Part model, mm, in its own coordinate system. A direction names the side the tool comes from. Round coordinates to 2 decimals unless told otherwise and drop trailing zeros. Order: outer loops, then holes, each group sorted by start corner. A loop starts at its lowest first (then second) coordinate and runs counter-clockwise, first axis right, second up. Notation, with made-up numbers: (-15.75, 66.5) - (2.25, 66.5) arc R35 cw to (2.25, 100.5) - close; hole circle Ø11 at (78, -14.5). An arc over 180 degrees is marked (long way). Answer as a JSON object with one key per item and string values.
```python
from build123d import *

# Parameters (mm, degrees)
SKETCH_1_W          = 33
SKETCH_1_H          = 62
EXTRUDE_1_DEPTH     = 8
SKETCH_2_W          = 15
SKETCH_2_H          = 10
CUT_EXTRUDE_1_DEPTH = 37.017356927
SKETCH_3_R          = 1.5
CUT_EXTRUDE_2_DEPTH = 37.017356927
SKETCH_4_R          = 1.5
CUT_EXTRUDE_3_DEPTH = 46.97825573
FILLET_2_R          = 1
SKETCH_5_R          = 1.5
CUT_EXTRUDE_4_DEPTH = 37.017356927
SKETCH_7_W          = 15
SKETCH_7_H          = 10
CUT_EXTRUDE_5_DEPTH = 37.017356927
FILLET_3_R          = 3
SKETCH_8_R          = 3.5
SKETCH_8_R_2        = 3
CUT_EXTRUDE_6_DEPTH = 3.5


with BuildPart() as part:
    # 草图1 → 凸台-拉伸1 (new body)
    with BuildSketch(Plane.XY):
        Rectangle(SKETCH_1_W, SKETCH_1_H)
    extrude(amount=EXTRUDE_1_DEPTH)

    # 草图2 → 切除-拉伸1 (cut, through all)
    with BuildSketch(Plane.XY.offset(8)):
        with Locations((0, 26)):
            Rectangle(SKETCH_2_W, SKETCH_2_H)
        with Locations((0, -26)):
            Rectangle(SKETCH_2_W, SKETCH_2_H)
    extrude(amount=-CUT_EXTRUDE_1_DEPTH, mode=Mode.SUBTRACT)

    # 草图3 → 切除-拉伸2 (cut, through all)
    with BuildSketch(Plane.XY.offset(8)):
        with Locations((11.5, 13)):
            Circle(SKETCH_3_R)
        with Locations((11.5, 21)):
            Circle(SKETCH_3_R)
        with Locations(Location((11.5, -21, 0), (0, 0, 180))):
            Circle(SKETCH_3_R)
        with Locations(Location((11.5, -13, 0), (0, 0, 180))):
            Circle(SKETCH_3_R)
        with Locations((-11.5, -13)):
            Circle(SKETCH_3_R)
        with Locations((-11.5, -21)):
            Circle(SKETCH_3_R)
        with Locations(Location((-11.5, 21, 0), (0, 0, 180))):
            Circle(SKETCH_3_R)
        with Locations(Location((-11.5, 13, 0), (0, 0, 180))):
            Circle(SKETCH_3_R)
    extrude(amount=-CUT_EXTRUDE_2_DEPTH, mode=Mode.SUBTRACT)

    # 草图4 → 切除-拉伸3 (cut, through all)
    with BuildSketch(Plane.ZY.offset(16.5)):
        with Locations((5, 27)):
            Circle(SKETCH_4_R)
        with Locations(Location((5, -27, 0), (0, 0, 180))):
            Circle(SKETCH_4_R)
    extrude(amount=-CUT_EXTRUDE_3_DEPTH, mode=Mode.SUBTRACT)

    # 圆角2
    fillet_2_edges = [part.edges().sort_by_distance(p)[0] for p in [
        (7.5, 21, 4),
        (-7.5, 21, 4),
        (-7.5, -21, 4),
        (7.5, -21, 4),
    ]]
    fillet(fillet_2_edges, radius=FILLET_2_R)

    # 草图5 → 切除-拉伸4 (cut, through all)
    with BuildSketch(Plane(origin=(0, 0, 0), x_dir=(-1, 0, 0), z_dir=(0, 0, -1))):
        Circle(SKETCH_5_R)
        with Locations((0, 18)):
            Circle(SKETCH_5_R)
        with Locations(Location((0, -18, 0), (0, 0, 180))):
            Circle(SKETCH_5_R)
    extrude(amount=-CUT_EXTRUDE_4_DEPTH, mode=Mode.SUBTRACT)

    # 草图7 → 切除-拉伸5 (cut, through all)
    with BuildSketch(Plane(origin=(0, 0, 0), x_dir=(-1, 0, 0), z_dir=(0, 0, -1))):
        with Locations((0, 9)):
            Rectangle(SKETCH_7_W, SKETCH_7_H)
        with Locations((0, -9)):
            Rectangle(SKETCH_7_W, SKETCH_7_H)
    extrude(amount=-CUT_EXTRUDE_5_DEPTH, mode=Mode.SUBTRACT)

    # 圆角3
    fillet_3_edges = [part.edges().sort_by_distance(p)[0] for p in [
        (-7.5, 14, 4),
        (-7.5, 4, 4),
        (7.5, 4, 4),
        (7.5, 14, 4),
        (7.5, -14, 4),
        (7.5, -4, 4),
        (-7.5, -4, 4),
        (-7.5, -14, 4),
    ]]
    fillet(fillet_3_edges, radius=FILLET_3_R)

    # 草图8 → 切除-拉伸6 (cut)
    with BuildSketch(Plane(origin=(0, 0, 0), x_dir=(-1, 0, 0), z_dir=(0, 0, -1))):
        with Locations((11.5, 21)):
            Circle(SKETCH_8_R)
        with Locations((-11.5, 21)):
            Circle(SKETCH_8_R)
        with Locations((-11.5, -21)):
            Circle(SKETCH_8_R)
        with Locations((11.5, -21)):
            Circle(SKETCH_8_R)
        Circle(SKETCH_8_R_2)
    extrude(amount=-CUT_EXTRUDE_6_DEPTH, mode=Mode.SUBTRACT)


solid = part.part
```
Item 1: Cut at B-B (y = 0). Write the cut outline in (x, z).
Taken from the geometry:
{"outline": "(-16.5, 0) - (-3, 0) - (-3, 3.5) - (-1.5, 3.5) - (-1.5, 8) - (-16.5, 8) - close; (1.5, 3.5) - (3, 3.5) - (3, 0) - (16.5, 0) - (16.5, 8) - (1.5, 8) - close"}
Item 2: Cut at C-C (y = 27). Write the cut outline in (x, z), plus the area to 3 significant figures.
Taken from the geometry:
{"outline": "(-16.5, 0) - (-7.5, 0) - (-7.5, 3.5) - (-16.5, 3.5) - close; (-16.5, 6.5) - (-7.5, 6.5) - (-7.5, 8) - (-16.5, 8) - close; (7.5, 0) - (16.5, 0) - (16.5, 3.5) - (7.5, 3.5) - close; (7.5, 6.5) - (16.5, 6.5) - (16.5, 8) - (7.5, 8) - close", "area": "90.0 mm2"}
Item 3: Cut at A-A (x = -11.5). State how many separate pieces and enclosed holes the cut face has, plus the area to 3 significant figures.
Taken from the geometry:
{"separate pieces": "5", "enclosed holes": "2", "area": "358 mm2"}
Item 4: Probe L1, parallel to Y at x = 0, z = 6.2; L2, parallel to Y at x = -11.5, z = 2.4; L3, parallel to Y at x = 11.5, z = 6.9. List the from-to ranges inside material, lowest first. Write a range as from..to.
Taken from the geometry:
{"L1": "-21..-19.5, -16.5..-14, -4..-1.5, 1.5..4, 14..16.5, 19.5..21", "L2": "-31..-24.5, -17.5..-14.5, -11.5..11.5, 14.5..17.5, 24.5..31", "L3": "-31..-22.5, -19.5..-14.5, -11.5..11.5, 14.5..19.5, 22.5..31"}
Item 5: Drop flat-ended pins along their axis: P1, Ø1.8, axis at x = -11.5, y = 13, coming from the +Z side; P2, Ø2.5, axis at x = 0.5, z = 2.5, coming from the +Y side; P3, Ø1.5, axis at x = -3.5, z = 7, coming from the -Y side. Give the stop position or say it passes through.
Taken from the geometry:
{"P1": "through", "P2": "y = 21", "P3": "y = -21"}
Item 6: Two-plate mould, pull along Y, no slides. Class faces 4 (the flat face through (0, -21, 4)), 5 (the flat face through (7.5, 26, 3)), 6 (the flat face through (7.5, -9, 4)): pulls with the +Y half, pulls with the -Y half, needs draft (parallel to the pull), parting line crosses it, or undercut.
Taken from the geometry:
{"face 4": "pulls with the -Y half", "face 5": "needs draft", "face 6": "undercut"}
Item 7: Tool access for faces 1 (the cylindrical face through (6.64, 13.1, 4.06)), 2 (the cylindrical face through (3, 0, 2)), 3 (the flat face through (-12, -31, 4)): list every direction of +Z, -Z, +X, -X, +Y, -Y with a clear straight run to the whole face (end or side of a thin tool).
Taken from the geometry:
{"face 1": "+Z, -Z", "face 2": "-Z", "face 3": "+Z, -Z, +X, -X, -Y"}
